Input: part model. Units: mm. Frame: model coordinates. Face numbers are marked on the shaded views. A direction names the side the tool comes from. Round coordinates to 2 decimals unless told otherwise and drop trailing zeros. Loops run counter-clockwise (first coordinate to the right, second up) from the corner with the lowest first, then second, coordinate; pieces in that order, holes last. Notation, with made-up numbers: (31.5, 50) -> (78.5, 50) arc R9 ccw to (78.5, 55) -> close; hole circle Ø11 at (64.5, 34). An arc over 180 degrees is marked (long way). Answer in a Markdown table with one row per item. Add a question column.
Q1. Section A-A, the plane x = 30. Output: boundary loops of the cut face in (y, z), and give its area (3 significant figures).
Q2. Reachability of the marked faces 1 and 2 from +Z, -Z, +X, -X, +Y, -Y: full face, straight path, thin tool, end or side. Return the list, or none.
Q3. Section B-B, the plane z = 8.5. Output: boundary loops of the cut face in (x, y).
Q4. Section D-D, the plane z = 15. Output: boundary loops of the cut face in (x, y), and give its area (3 significant figures).
Q5. Ray query, L1, parallel to X at y = 0.25, z = 7.25; L2, parallel to X at y = 14, z = 2.25; L3, parallel to Y at x = -10, z = 16. Return the intervals inside material, ascending. Write a range as from..to.
Q6. Mould query, pull axis Y, two halves, no side actions, for the marked faces 3, 4, 5 and 6. Classes: pulls with the +Y half, pulls with the -Y half, needs draft (parallel to the pull), parting line crosses it, or undercut.
Q7. Pin query (flat end, axial travel): pin 1 (3.5 mm diameter, centred on x = -8, y = 1, fed in from -Z); pin 2 (6.5 mm diameter, centred on x = 30, y = -5, fed in from -Z). Return the tip coordinate at first contact, or that it passes through.
Q8. Section C-C, the plane y = -5. Output: boundary loops of the cut face in (x, z), and give its area (3 significant figures).
```python
from build123d import *

# Parameters (mm, degrees)
SKETCH_1_W          = 90
SKETCH_1_H          = 30
EXTRUDE_1_DEPTH     = 20
SKETCH_3_R          = 6
CUT_EXTRUDE_1_DEPTH = 12
SKETCH_4_R          = 3
CUT_EXTRUDE_2_DEPTH = 49.928519291
SKETCH_5_W          = 8
SKETCH_5_H          = 5
CUT_EXTRUDE_3_DEPTH = 58.662812973
SKETCH_6_R          = 4
CUT_EXTRUDE_4_DEPTH = 52.478150705


with BuildPart() as part:
    # Эскиз1 → Бобышка-Вытянуть1 (new body)
    with BuildSketch(Plane.XY):
        Rectangle(SKETCH_1_W, SKETCH_1_H)
    extrude(amount=EXTRUDE_1_DEPTH)

    # Эскиз2 → Вырез-Повернуть1 (revolve, cut)
    with BuildSketch(Plane(origin=(0, 0, 0), x_dir=(1, 0, 0), z_dir=(0, 1, 0)), mode=Mode.PRIVATE) as cut_revolve_1_sk:
        Polygon((-30, 0), (-26, 0), (-26, -10), (-30, -14), align=None)
    revolve(cut_revolve_1_sk.sketch.rotate(Axis((-30, 0, 0), (0, 0, 1)), 180), axis=Axis((-30, 0, 0), (0, 0, 1)), mode=Mode.SUBTRACT)

    # Эскиз3 → Вырез-Вытянуть1 (cut)
    with BuildSketch(Plane(origin=(0, 0, 0), x_dir=(-1, 0, 0), z_dir=(0, 0, -1))):
        with Locations((10, 0)):
            Circle(SKETCH_3_R)
    extrude(amount=-CUT_EXTRUDE_1_DEPTH, mode=Mode.SUBTRACT)

    # Эскиз4 → Вырез-Вытянуть2 (cut, through all)
    with BuildSketch(Plane(origin=(0, 0, 12), x_dir=(-1, 0, 0), z_dir=(0, 0, -1))):
        with Locations((10, 0)):
            Circle(SKETCH_4_R)
    extrude(amount=-CUT_EXTRUDE_2_DEPTH, mode=Mode.SUBTRACT)

    # Эскиз5 → Вырез-Вытянуть3 (cut, through all)
    with BuildSketch(Plane(origin=(0, 15, 0), x_dir=(1, 0, 0), z_dir=(0, 1, 0))):
        with Locations((11, -2.5)):
            Rectangle(SKETCH_5_W, SKETCH_5_H)
    extrude(amount=-CUT_EXTRUDE_3_DEPTH, mode=Mode.SUBTRACT)

    # Эскиз6 → Вырез-Вытянуть4 (cut, through all)
    with BuildSketch(Plane(origin=(0, 0, 0), x_dir=(-1, 0, 0), z_dir=(0, 0, -1))):
        with Locations((-30, -5)):
            Circle(SKETCH_6_R)
    extrude(amount=-CUT_EXTRUDE_4_DEPTH, mode=Mode.SUBTRACT)


solid = part.part
```
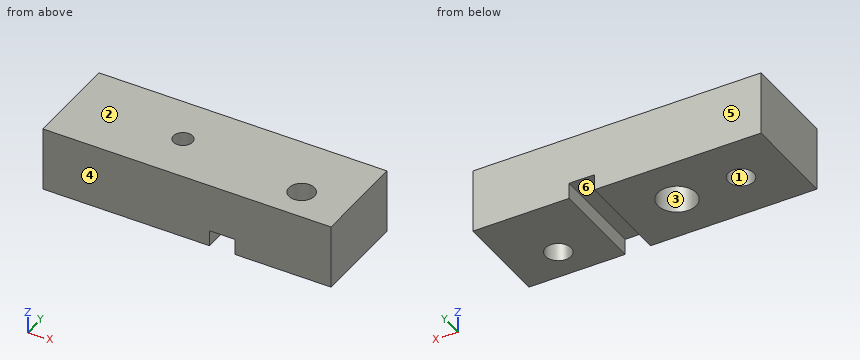
Answer block:
| question | item | result |
|---|---|---|
| 1 | outline | (-15, 0) -> (-9, 0) -> (-9, 20) -> (-15, 20) -> close; (-1, 0) -> (15, 0) -> (15, 20) -> (-1, 20) -> close |
| 1 | area | 440 mm^2 |
| 2 | face 1 | -Z |
| 2 | face 2 | +Z, +X, -X, +Y, -Y |
| 3 | outline | (-45, -15) -> (45, -15) -> (45, 15) -> (-45, 15) -> close; hole circle Ø8 at (-30, 0); hole circle Ø12 at (-10, 0); hole circle Ø8 at (30, -5) |
| 4 | outline | (-45, -15) -> (45, -15) -> (45, 15) -> (-45, 15) -> close; hole circle Ø6 at (-10, 0); hole circle Ø8 at (30, -5) |
| 4 | area | 2,620 mm^2 |
| 5 | L1 | -45..-33.99, -26.01..-15.99, -4.01..45 |
| 5 | L2 | -45..7, 15..45 |
| 5 | L3 | -15..-3, 3..15 |
| 6 | face 3 | undercut |
| 6 | face 4 | pulls with the -Y half |
| 6 | face 5 | pulls with the +Y half |
| 6 | face 6 | needs draft |
| 7 | pin 1 | z = 12 |
| 7 | pin 2 | through |
| 8 | outline | (-45, 0) -> (-13.32, 0) -> (-13.32, 12) -> (-6.68, 12) -> (-6.68, 0) -> (7, 0) -> (7, 5) -> (15, 5) -> (15, 0) -> (26, 0) -> (26, 20) -> (-45, 20) -> close; (34, 0) -> (45, 0) -> (45, 20) -> (34, 20) -> close |
| 8 | area | 1,520 mm^2 |
